Can you work these out from the model? Positions are in its coordinate system, mm. A direction names the side the tool comes from. Coordinates: 2 decimals unless noted, no trailing zeros. Write each loop counter-clockwise with the first axis right and the second up, starting at its lowest first coordinate (ties: lowest second). Pieces come first, ordered by that corner, then holes. Notation, with made-up numbers: (-24.5, 6.5) -> (6.5, 6.5) arc R16 ccw to (6.5, 16.5) -> close; hole circle Ø6 at (63, 44). An arc over 180 degrees is marked (long way). Use one line per item in the form item = value.
Autodesk Inventor part; units mm, degrees
ref_plane "YZ Plane" through (0, 0, 0) normal (1, 0, 0) x (0, 1, 0)
ref_plane "XZ Plane" through (0, 0, 0) normal (0, 1, 0) x (-1, 0, 0)
ref_plane "XY Plane" through (0, 0, 0) normal (0, 0, 1) x (1, 0, 0)
sketch "Sketch1" plane through (0, 0, 0) normal (0, 1, 0) x (-1, 0, 0)
  circle A0 centre (0, 0) radius 3
  circle A1 centre (0, 0) radius 4.375
  dimension "d0" = 6
  dimension "d1" = 8.75
extrude "Extrusion1" add sketch "Sketch1" along normal blind 2.7
sketch "Sketch2" plane through (0, 2.7, 0) normal (0, 1, 0) x (1, 0, 0)
  circle A0 centre (0, 0) radius 3
  circle A1 centre (0, 0) radius 4.375
extrude "Extrusion2" add sketch "Sketch2" along normal blind 0.6 contours A0 | A1
sketch "Sketch3" plane through (0, 3.3, 0) normal (0, 1, 0) x (1, 0, 0)
  circle A0 centre (0, 0) radius 12.5
  dimension "d9" = 25
extrude "Extrusion3" add sketch "Sketch3" along normal blind 2.4
properties part number "Estella Servo1"
Q1. Suppose I cut it at C-C (x = -8.25). Write out the boundary of the cut face in (y, z).
Return value:
outline = (3.3, -9.39) -> (5.7, -9.39) -> (5.7, 9.39) -> (3.3, 9.39) -> close
Q2. Suppose I cut it at B-B (y = 4.1). Write out the boundary of the cut face in (x, z).
Return value:
outline = circle Ø25 at (0, 0)
Q3. Suppose I cut it at A-A (z = -4). Write out the boundary of the cut face in (x, y), then the cut area to 3 significant figures.
Return value:
outline = (-11.84, 3.3) -> (-1.77, 3.3) -> (-1.77, 0) -> (1.77, 0) -> (1.77, 3.3) -> (11.84, 3.3) -> (11.84, 5.7) -> (-11.84, 5.7) -> close
area = 68.5 mm2
Q4. For faces 1 (the cylindrical face through (3, 1, 0)), 2 (the flat face through (1, 0, -3)), which set-ups out of +Z, -Z, +X, -X, +Y, -Y let a thin tool reach every point of the face, with its end or its side?
Return value:
face_1 = -Y
face_2 = +Z, -Z, +X, -X, -Y
Q5. Will these pins go through, and if not, where does the flat tip stop? pin 1 (2 mm diameter, centred on x = -9.5, y = 2, fed in from -Z); pin 2 (2 mm diameter, centred on y = 1.5, z = -4, fed in from -X); pin 3 (3 mm diameter, centred on x = 0.5, z = -0.5, fed in from -Y); pin 4 (1 mm diameter, centred on y = 5, z = 9, fed in from -X).
Return value:
pin_1 = through
pin_2 = -3.18
pin_3 = 2.7
pin_4 = -9.17
Q6. If I drill on line 1 (Z direction, x = 0, y = 0.65) (3 decimals); line 2 (Y direction, x = -6.25, z = 0.5); line 3 (Y direction, x = -0.75, z = -1), over which ranges is the centre line in solid material (lowest first)? Write a range as from..to.
Return value:
line_1 = -4.375..-3, 3..4.375
line_2 = 3.3..5.7
line_3 = 2.7..5.7
Q7. Thinking about a two-plate mould opening in Z: for faces 3 (the cylindrical face through (11.923, 4.483, 3.755)), 4 (the flat face through (0, 3.3, 5)), 5 (the flat face through (0, 2.7, 0)), which applies, released by +Z, released by -Z, zero draft, split by the parting line, or undercut?
Return value:
face_3 = split by the parting line
face_4 = zero draft
face_5 = undercut
Q8. Suppose I cut it at D-D (z = -0.75). Write out the boundary of the cut face in (x, y), then the cut area to 3 significant figures.
Return value:
outline = (-12.48, 3.3) -> (-4.31, 3.3) -> (-4.31, 0) -> (-2.9, 0) -> (-2.9, 2.7) -> (2.9, 2.7) -> (2.9, 0) -> (4.31, 0) -> (4.31, 3.3) -> (12.48, 3.3) -> (12.48, 5.7) -> (-12.48, 5.7) -> close
area = 72.7 mm2
